```python
from build123d import *
from OCP.BRepFilletAPI import BRepFilletAPI_MakeChamfer

# Parameters (mm, degrees)
BOSS_EXTRUDE1_DEPTH = 50
SKETCH5_W           = 63
SKETCH5_H           = 50
BOSS_EXTRUDE2_DEPTH = 1.6
SKETCH9_W           = 10
SKETCH9_H           = 40
CUT_EXTRUDE4_DEPTH  = 1.5
CHAMFER4_SIZE       = 1.5
CHAMFER6_SIZE       = 0.8
CHAMFER6_SIZE2      = 0.738449877
CHAMFER7_SIZE       = 0.8
CHAMFER7_SIZE2      = 0.880050294
CHAMFER7_SIZE2_2    = 0.59857957
FILLET1_R           = 7
CHAMFER10_SIZE      = 1.5
CUT_EXTRUDE5_REACH  = 74.773
CUT_EXTRUDE6_DEPTH  = 1.6


with BuildPart() as part:
    # Sketch1 → Boss-Extrude1 (new body)
    with BuildSketch(Plane.XY):
        Polygon((-32.16425811, 32.5), (-27.555232111, 32.5), (-30.546782223, 38.65618727), (-28.747926936, 39.530326652), (-25.331595762, 32.5), (-25.331595762, 30.5), (-30.331595762, 30.5), (-33, 0), (0, 0), (33, 0), (30.331595762, 30.5), (25.331595762, 30.5), (25.331595762, 32.5), (28.747926936, 39.530326652), (30.546782223, 38.65618727), (27.555232111, 32.5), (32.16425811, 32.5), (35.182617002, -2), (0, -2), (-35.182617002, -2), align=None)
    extrude(amount=BOSS_EXTRUDE1_DEPTH)

    # Sketch5 → Boss-Extrude2 (add)
    with BuildSketch(Plane.XZ.offset(2)):
        with Locations((0, 25)):
            Rectangle(SKETCH5_W, SKETCH5_H)
    extrude(amount=BOSS_EXTRUDE2_DEPTH)

    # Sketch9 → Cut-Extrude4 (cut)
    with BuildSketch(Plane(origin=(0, 0, 0), x_dir=(1, 0, 0), z_dir=(0, 1, 0))):
        with Locations((0, -25)):
            Rectangle(SKETCH9_W, SKETCH9_H)
    extrude(amount=-CUT_EXTRUDE4_DEPTH, mode=Mode.SUBTRACT)

    # Chamfer4
    chamfer4_edges = [part.edges().sort_by_distance(p)[0] for p in [
        (0, 0, 45),
        (-5, 0, 25),
        (0, 0, 5),
        (5, 0, 25),
    ]]
    chamfer(chamfer4_edges, length=CHAMFER4_SIZE - 0.0001)  # a hair under: the kernel refuses the full size

    # Chamfer6: one chamfer whose edges measure the first distance from different faces: ONE call of the kernel's chamfer builder (chamfer() names one face for all edges)
    chamfer6_edges_1 = [part.edges().sort_by_distance(p)[0] for p in [
        (-33, 0, 25),
    ]]
    chamfer6_side_1 = [part.faces().sort_by_distance(p)[0] for p in [
        (0, 0, 47.327909662),
    ]]
    chamfer6_edges_2 = [part.edges().sort_by_distance(p)[0] for p in [
        (33, 0, 25),
    ]]
    chamfer6_side_2 = [part.faces().sort_by_distance(p)[0] for p in [
        (31.665797881, 15.25, 25),
    ]]
    chamfer6_edges_3 = [part.edges().sort_by_distance(p)[0] for p in [
        (35.182617002, -2, 25),
    ]]
    chamfer6_side_3 = [part.faces().sort_by_distance(p)[0] for p in [
        (33.341308501, -2, 25),
    ]]
    chamfer6_edges_4 = [part.edges().sort_by_distance(p)[0] for p in [
        (-35.182617002, -2, 25),
    ]]
    chamfer6_side_4 = [part.faces().sort_by_distance(p)[0] for p in [
        (-33.673437556, 15.25, 25),
    ]]
    chamfer6 = BRepFilletAPI_MakeChamfer(part.part.solid().wrapped)
    for e in chamfer6_edges_1:
        chamfer6.Add(CHAMFER6_SIZE, CHAMFER6_SIZE2, e.wrapped, chamfer6_side_1[0].wrapped)  # the first distance lies on this face
    for e in chamfer6_edges_2:
        chamfer6.Add(CHAMFER6_SIZE, CHAMFER6_SIZE2, e.wrapped, chamfer6_side_2[0].wrapped)  # the first distance lies on this face
    for e in chamfer6_edges_3:
        chamfer6.Add(CHAMFER6_SIZE, CHAMFER6_SIZE2, e.wrapped, chamfer6_side_3[0].wrapped)  # the first distance lies on this face
    for e in chamfer6_edges_4:
        chamfer6.Add(CHAMFER6_SIZE, CHAMFER6_SIZE2, e.wrapped, chamfer6_side_4[0].wrapped)  # the first distance lies on this face
    add(Compound.cast(chamfer6.Shape()), mode=Mode.REPLACE)

    # Chamfer7: one chamfer whose edges measure the first distance from different faces: ONE call of the kernel's chamfer builder (chamfer() names one face for all edges)
    chamfer7_edges_1 = [part.edges().sort_by_distance(p)[0] for p in [
        (-30.331595762, 30.5, 25),
    ]]
    chamfer7_side_1 = [part.faces().sort_by_distance(p)[0] for p in [
        (-31.633617807, 15.617819926, 25),
    ]]
    chamfer7_edges_2 = [part.edges().sort_by_distance(p)[0] for p in [
        (30.331595762, 30.5, 25),
    ]]
    chamfer7_side_2 = [part.faces().sort_by_distance(p)[0] for p in [
        (27.831595762, 30.5, 25),
    ]]
    chamfer7_edges_3 = [part.edges().sort_by_distance(p)[0] for p in [
        (27.555232111, 32.5, 25),
    ]]
    chamfer7_side_3 = [part.faces().sort_by_distance(p)[0] for p in [
        (29.859745111, 32.5, 25),
    ]]
    chamfer7_edges_4 = [part.edges().sort_by_distance(p)[0] for p in [
        (32.16425811, 32.5, 25),
    ]]
    chamfer7_side_4 = [part.faces().sort_by_distance(p)[0] for p in [
        (33.641257483, 15.617819926, 25),
    ]]
    chamfer7_edges_5 = [part.edges().sort_by_distance(p)[0] for p in [
        (-32.16425811, 32.5, 25),
    ]]
    chamfer7_side_5 = [part.faces().sort_by_distance(p)[0] for p in [
        (-29.859745111, 32.5, 25),
    ]]
    chamfer7_edges_6 = [part.edges().sort_by_distance(p)[0] for p in [
        (-27.555232111, 32.5, 25),
    ]]
    chamfer7_side_6 = [part.faces().sort_by_distance(p)[0] for p in [
        (-29.051007167, 35.578093635, 25),
    ]]
    chamfer7 = BRepFilletAPI_MakeChamfer(part.part.solid().wrapped)
    for e in chamfer7_edges_1:
        chamfer7.Add(CHAMFER7_SIZE, CHAMFER7_SIZE2, e.wrapped, chamfer7_side_1[0].wrapped)  # the first distance lies on this face
    for e in chamfer7_edges_2:
        chamfer7.Add(CHAMFER7_SIZE, CHAMFER7_SIZE2, e.wrapped, chamfer7_side_2[0].wrapped)  # the first distance lies on this face
    for e in chamfer7_edges_3:
        chamfer7.Add(CHAMFER7_SIZE, CHAMFER7_SIZE2_2, e.wrapped, chamfer7_side_3[0].wrapped)  # the first distance lies on this face
    for e in chamfer7_edges_4:
        chamfer7.Add(CHAMFER7_SIZE, CHAMFER7_SIZE2, e.wrapped, chamfer7_side_4[0].wrapped)  # the first distance lies on this face
    for e in chamfer7_edges_5:
        chamfer7.Add(CHAMFER7_SIZE, CHAMFER7_SIZE2, e.wrapped, chamfer7_side_5[0].wrapped)  # the first distance lies on this face
    for e in chamfer7_edges_6:
        chamfer7.Add(CHAMFER7_SIZE, CHAMFER7_SIZE2_2, e.wrapped, chamfer7_side_6[0].wrapped)  # the first distance lies on this face
    add(Compound.cast(chamfer7.Shape()), mode=Mode.REPLACE)

    # Fillet1
    fillet1_edges = [part.edges().sort_by_distance(p)[0] for p in [
        (-31.5, -2.8, 0),
        (31.5, -2.8, 0),
        (31.5, -2.8, 50),
        (-31.5, -2.8, 50),
    ]]
    fillet(fillet1_edges, radius=FILLET1_R)

    # Chamfer10
    chamfer10_edges = [part.edges().sort_by_distance(p)[0] for p in [
        (-31.5, -3.6, 25),
        (0, -3.6, 50),
        (0, -3.6, 0),
        (31.5, -3.6, 25),
        (29.449747468, -3.6, 47.949747468),
        (29.449747468, -3.6, 2.050252532),
        (-29.449747468, -3.6, 2.050252532),
        (-29.449747468, -3.6, 47.949747468),
    ]]
    chamfer(chamfer10_edges, length=CHAMFER10_SIZE)

    # Sketch15 → Cut-Extrude5 (cut, up to next)
    with BuildSketch(Plane(origin=(0, 0, 0), x_dir=(1, 0, 0), z_dir=(0, 1, 0)), mode=Mode.PRIVATE) as cut_extrude5_sk1:
        with BuildLine():
            Line((21.475016583, -42.866268583), (20.428249938, -41.819501939))
            ThreePointArc((20.428249938, -41.819501939), (16.022847213, -33.655561292), (24.186787861, -38.060964016))
            Line((24.186787861, -38.060964016), (25.233554505, -39.107730661))
            ThreePointArc((25.233554505, -39.107730661), (26.877324102, -44.51003818), (21.475016583, -42.866268583))
        make_face()
    cut_extrude5_tool1 = extrude(cut_extrude5_sk1.sketch, amount=-CUT_EXTRUDE5_REACH, mode=Mode.PRIVATE) & part.part
    # Sketch15 → Cut-Extrude5 (cut, up to next)
    with BuildSketch(Plane(origin=(0, 0, 0), x_dir=(1, 0, 0), z_dir=(0, 1, 0)), mode=Mode.PRIVATE) as cut_extrude5_sk2:
        with BuildLine():
            Line((-25.185393692, -39.138763585), (-24.139916413, -38.090709162))
            ThreePointArc((-24.139916413, -38.090709162), (-15.98140501, -33.675259948), (-20.37675457, -41.844617469))
            Line((-20.37675457, -41.844617469), (-21.422231849, -42.892671893))
            ThreePointArc((-21.422231849, -42.892671893), (-26.822511792, -44.543090495), (-25.185393692, -39.138763585))
        make_face()
    cut_extrude5_tool2 = extrude(cut_extrude5_sk2.sketch, amount=-CUT_EXTRUDE5_REACH, mode=Mode.PRIVATE) & part.part
    # Sketch15 → Cut-Extrude5 (cut, up to next)
    with BuildSketch(Plane(origin=(0, 0, 0), x_dir=(1, 0, 0), z_dir=(0, 1, 0)), mode=Mode.PRIVATE) as cut_extrude5_sk3:
        with BuildLine():
            Line((25.233554505, -10.892269339), (24.186787861, -11.939035984))
            ThreePointArc((24.186787861, -11.939035984), (16.022847213, -16.344438708), (20.428249938, -8.180498061))
            Line((20.428249938, -8.180498061), (21.475016583, -7.133731417))
            ThreePointArc((21.475016583, -7.133731417), (26.877324102, -5.48996182), (25.233554505, -10.892269339))
        make_face()
    cut_extrude5_tool3 = extrude(cut_extrude5_sk3.sketch, amount=-CUT_EXTRUDE5_REACH, mode=Mode.PRIVATE) & part.part
    # Sketch15 → Cut-Extrude5 (cut, up to next)
    with BuildSketch(Plane(origin=(0, 0, 0), x_dir=(1, 0, 0), z_dir=(0, 1, 0)), mode=Mode.PRIVATE) as cut_extrude5_sk4:
        with BuildLine():
            Line((-21.422231849, -7.107328107), (-20.37675457, -8.155382531))
            ThreePointArc((-20.37675457, -8.155382531), (-15.98140501, -16.324740052), (-24.139916413, -11.909290838))
            Line((-24.139916413, -11.909290838), (-25.185393692, -10.861236415))
            ThreePointArc((-25.185393692, -10.861236415), (-26.822511792, -5.456909505), (-21.422231849, -7.107328107))
        make_face()
    cut_extrude5_tool4 = extrude(cut_extrude5_sk4.sketch, amount=-CUT_EXTRUDE5_REACH, mode=Mode.PRIVATE) & part.part
    add(cut_extrude5_tool1.solids().sort_by_distance((21.014912, 0, 38.647626))[0], mode=Mode.SUBTRACT)
    add(cut_extrude5_tool2.solids().sort_by_distance((-20.96732, 0, 38.673466))[0], mode=Mode.SUBTRACT)
    add(cut_extrude5_tool3.solids().sort_by_distance((21.014912, 0, 11.352374))[0], mode=Mode.SUBTRACT)
    add(cut_extrude5_tool4.solids().sort_by_distance((-20.96732, 0, 11.326534))[0], mode=Mode.SUBTRACT)

    # Sketch16 → Cut-Extrude6 (cut)
    with BuildSketch(Plane(origin=(0, 0, 0), x_dir=(1, 0, 0), z_dir=(0, 1, 0))):
        with BuildLine():
            Line((-15.951616609, -40.543181032), (-21.113676241, -45.71796535))
            ThreePointArc((-21.113676241, -45.71796535), (-28.002957525, -45.726446075), (-28.011438251, -38.837164791))
            Line((-28.011438251, -38.837164791), (-22.849378618, -33.662380473))
            ThreePointArc((-22.849378618, -33.662380473), (-15.960097334, -33.653899748), (-15.951616609, -40.543181032))
        make_face()
        with BuildLine():
            Line((-15.951616609, -9.456818968), (-21.113676241, -4.28203465))
            ThreePointArc((-21.113676241, -4.28203465), (-28.002957525, -4.273553925), (-28.011438251, -11.162835209))
            Line((-28.011438251, -11.162835209), (-22.849378618, -16.337619527))
            ThreePointArc((-22.849378618, -16.337619527), (-15.960097334, -16.346100252), (-15.951616609, -9.456818968))
        make_face()
        with BuildLine():
            Line((15.951616609, -40.543181032), (21.113676241, -45.71796535))
            ThreePointArc((21.113676241, -45.71796535), (28.002957525, -45.726446075), (28.011438251, -38.837164791))
            Line((28.011438251, -38.837164791), (22.849378618, -33.662380473))
            ThreePointArc((22.849378618, -33.662380473), (15.960097334, -33.653899748), (15.951616609, -40.543181032))
        make_face()
        with BuildLine():
            Line((15.951616609, -9.456818968), (21.113676241, -4.28203465))
            ThreePointArc((21.113676241, -4.28203465), (28.002957525, -4.273553925), (28.011438251, -11.162835209))
            Line((28.011438251, -11.162835209), (22.849378618, -16.337619527))
            ThreePointArc((22.849378618, -16.337619527), (15.960097334, -16.346100252), (15.951616609, -9.456818968))
        make_face()
    extrude(amount=-CUT_EXTRUDE6_DEPTH, mode=Mode.SUBTRACT)


solid = part.part
```
The model under review builds one solid part; all positions refer to its coordinate system, in mm. A direction names the side the tool comes from. Round coordinates to 2 decimals unless told otherwise and drop trailing zeros. Write each loop counter-clockwise with the first axis right and the second up, starting at its lowest first coordinate (ties: lowest second). Pieces come first, ordered by that corner, then holes.
(1) We need section C-C on y = 2. Give the boundary of the cut face in (x, z).
(2) Mouldability with a two-part tool opening along Y and no side actions: class faces 1 (the flat face through (-25.47, -0.79, 36.29)), 2 (the flat face through (-33.697, 14.98, 24.65)), 3 (the cylindrical face through (-16.11, -2.59, 33.55)) as +Y half, -Y half, draft (parallel to the pull), parting line (faces both ways), or undercut.
(3) Wall thickness on L1, parallel to Y at x = -30, z = 14; L2, parallel to Y at x = -16, z = 18; L3, parallel to Y at x = 3, z = 44.5: over which ranges is each line inside the solid? List them lowest first.
(4) Machinability: for faces 4 (the flat face through (21, -1.6, 43)), 5 (the cylindrical face through (-26.753, -2.586, 44.61)), 6 (the flat face through (27, 30.5, 25)), 7 (the flat face through (-0.1, -0.8, 4.3)), 8 (the flat face through (25.332, 31, 25)), which of the approach directions +Z, -Z, +X, -X, +Y, -Y give a long, thin tool a straight path to every point of the face, cutting with its end or side? Answer none if there is none.
(5) Insertion check: pin 1 (4 mm diameter, centred on y = 12, z = 36.5, fed in from -X); pin 2 (1.5 mm diameter, centred on x = 8, z = 10.5, fed in from +Y); pin 3 (4 mm diameter, centred on x = 24.61, z = 7.75, fed in from +Y); pin 4 (5 mm diameter, centred on x = 22.5, z = 42, fed in from -Y). Each pin has a flat end and moves straight along its axis. Give the tip position at first contact, or say it passes through.
(6) We need section A-A on y = 36.5. Give the boundary of the cut face in (x, z).
Findings below:
1. outline: (-34.83, 0) - (-32.83, 0) - (-32.83, 50) - (-34.83, 50) - close; (32.83, 0) - (34.83, 0) - (34.83, 50) - (32.83, 50) - close
2. face 1: undercut
2. face 2: +Y half
2. face 3: draft
3. L1: y = -3.6 to 0, 30.04 to 32.5, 37.53 to 38.92
3. L2: y = -3.6 to 0
3. L3: y = -3.6 to -1.5
4. face 4: none
4. face 5: -Y
4. face 6: +Z, -Z
4. face 7: +Y
4. face 8: +Z, -Z, +Y
5. pin 1: stops at x = -34.13
5. pin 2: stops at y = 0
5. pin 3: stops at y = 35.13
5. pin 4: stops at y = -3.6
6. outline: (-29.5, 0) - (-27.28, 0) - (-27.28, 50) - (-29.5, 50) - close; (27.28, 0) - (29.5, 0) - (29.5, 50) - (27.28, 50) - close
